Input: part model. Units: mm. Frame: model coordinates. A direction names the side the tool comes from. Coordinates: 2 decimals unless noted, no trailing zeros. Write each loop counter-clockwise with the first axis right and the second up, starting at its lowest first coordinate (ties: lowest second). Pieces come first, ordered by that corner, then holes. Notation, with made-up numbers: (30, -13.5) - (36, -13.5) arc R29 ccw to (36, 25.5) - close; hole circle Ø5 at (14, 77). An arc over 180 degrees is marked (long way). Put each result on its own line as item: value. Start each with the question number.
1. Pin query (flat end, axial travel): pin 1 (1.5 mm diameter, centred on x = 47, z = 41, fed in from +Y); pin 2 (3 mm diameter, centred on x = -53.5, z = 33, fed in from -Y); pin 3 (1.5 mm diameter, centred on x = -37.5, z = 46, fed in from -Y); pin 4 (3 mm diameter, centred on x = -49, z = 54.5, fed in from +Y). Return the tip coordinate at first contact, or that it passes through.
2. Cut plane A-A, the plane y = -168.5. Return loops of the section in (x, z), and give its area (3 significant figures).
3. Access query for faces 5 (the cylindrical face through (-5.506, -100.178, 24.796)), 6 (the conical face through (-10.276, 2.846, -32.631)). Directions: +Z, -Z, +X, -X, +Y, -Y. A direction counts if a zero-diameter tool reaches every point of the face in a straight line with its end or side. Return the directions, or none.
4. Pull-direction query (X, two-part tool) for faces 1 (the conical face through (1.39, -221.71, 4.41)), 2 (the conical face through (26.66, 2.21, 5.92)), 3 (the flat face through (-16, 45.488, 64)), 4 (the cylindrical face through (-6.883, -100.178, 30.995)); classes: released by +X, released by -X, zero draft, split by the parting line, or undercut.
5. Line query: line 1 (Z direction, x = 0, y = -141); line 2 (Z direction, x = 23.5, y = -77). Output: solid intervals per line, ascending.
from build123d import *

# Parameters (mm, degrees)
SKETCH2_R           = 31.75
SKETCH2_R_2         = 25.4
BOSS_EXTRUDE1_DEPTH = 254
SKETCH5_R           = 46.805948237
CUT_EXTRUDE1_DEPTH  = 50.8


with BuildPart() as part:
    # Sketch2 → Boss-Extrude1 (new body)
    with BuildSketch(Plane(origin=(0, 0, 0), x_dir=(1, 0, 0), z_dir=(0, 1, 0))):
        Circle(SKETCH2_R)
        Circle(SKETCH2_R_2, mode=Mode.SUBTRACT)
    extrude(amount=-BOSS_EXTRUDE1_DEPTH)

    # Sketch4 → Revolve1 (revolve)
    with BuildSketch(Plane(origin=(0, 0, 0), x_dir=(0, 0, -1), z_dir=(1, 0, 0))):
        Polygon((31.75, 0), (71.093054088, 45.488426276), (64.743054088, 45.488426276), (25.4, 0), align=None)
    revolve(axis=Axis((0, 0, 0), (0, 1, 0)))

    # Sketch5 → Cut-Extrude1 (cut)
    with BuildSketch(Plane.XZ.offset(254)):
        Circle(SKETCH5_R)
    extrude(amount=-CUT_EXTRUDE1_DEPTH, mode=Mode.SUBTRACT)

    # Sketch6 → Revolve2 (revolve)
    with BuildSketch(Plane(origin=(0, 0, 0), x_dir=(0, 0, -1), z_dir=(1, 0, 0))):
        Polygon((-31.75, -203.2), (-25.4, -203.2), (-0.675857916, -225.226857467), (-1.351715832, -227.518627335), align=None)
    revolve(axis=Axis((0, -254, 0), (0, 1, 0)))


solid = part.part
Report:
1. pin 1: stops at y = 43.61
1. pin 2: stops at y = 34.23
1. pin 3: stops at y = 31.04
1. pin 4: passes through
2. outline: circle Ø63.5 at (0, 0); hole circle Ø50.8 at (0, 0)
2. area: 1,140 mm^2
3. face 5: +Y
3. face 6: -Y
4. face 1: undercut
4. face 2: undercut
4. face 3: zero draft
4. face 4: split by the parting line
5. line 1: z = -31.75 to -25.4, 25.4 to 31.75
5. line 2: z = -21.35 to -9.64, 9.64 to 21.35
